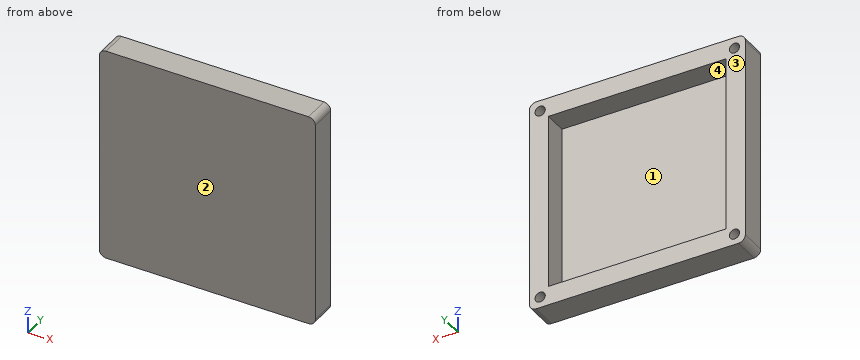
from build123d import *

# Parameters (mm, degrees)
SKETCH1_W           = 63.5
SKETCH1_H           = 63.5
BOSS_EXTRUDE1_DEPTH = 7.8
SKETCH2_W           = 52.2
SKETCH2_H           = 52.2
CUT_EXTRUDE1_DEPTH  = 6.8
SKETCH3_R           = 1.5
CUT_EXTRUDE2_DEPTH  = 7.5
FILLET1_R           = 2


with BuildPart() as part:
    # Sketch1 → Boss-Extrude1 (new body)
    with BuildSketch(Plane(origin=(0, 0, 0), x_dir=(1, 0, 0), z_dir=(0, 1, 0))):
        with Locations((31.75, 31.75)):
            Rectangle(SKETCH1_W, SKETCH1_H)
    extrude(amount=BOSS_EXTRUDE1_DEPTH)

    # Sketch2 → Cut-Extrude1 (cut)
    with BuildSketch(Plane(origin=(0, 7.8, 0), x_dir=(1, 0, 0), z_dir=(0, 1, 0))):
        with Locations((31.75, 31.75)):
            Rectangle(SKETCH2_W, SKETCH2_H)
    extrude(amount=-CUT_EXTRUDE1_DEPTH, mode=Mode.SUBTRACT)

    # Sketch3 → Cut-Extrude2 (cut)
    with BuildSketch(Plane(origin=(0, 7.8, 0), x_dir=(1, 0, 0), z_dir=(0, 1, 0))):
        with Locations(Location((3.2, 3.2, 0), (0, 0, 270))):
            Circle(SKETCH3_R)
        with Locations(Location((3.2, 60.3, 0), (0, 0, 270))):
            Circle(SKETCH3_R)
        with Locations(Location((60.3, 60.3, 0), (0, 0, 270))):
            Circle(SKETCH3_R)
        with Locations(Location((60.3, 3.2, 0), (0, 0, 270))):
            Circle(SKETCH3_R)
    extrude(amount=-CUT_EXTRUDE2_DEPTH, mode=Mode.SUBTRACT)

    # Fillet1
    fillet1_edges = [part.edges().sort_by_distance(p)[0] for p in [
        (0, 3.9, -63.5),
        (63.5, 3.9, -63.5),
        (63.5, 3.9, 0),
        (0, 3.9, 0),
    ]]
    fillet(fillet1_edges, radius=FILLET1_R)


solid = part.part
Build history of the part. All positions in model axes, mm. Face numbers are marked on the shaded views. A direction names the side the tool comes from. Coordinates: 2 decimals unless noted, no trailing zeros. Order: outer loops, then holes, each group sorted by start corner. A loop starts at its lowest first (then second) coordinate and runs counter-clockwise, first axis right, second up. Notation, with made-up numbers: (35, -21.75) - (42, -21.75) arc R20 ccw to (42, -2.75) - close; hole circle Ø3 at (45, -13). An arc over 180 degrees is marked (long way). Write item = value, one per line. Start each with the question number.
1) Saw through at A-A on z = -22.5. Write the cut outline in (x, y), then the cut area to 3 significant figures.
2) Flat gauge pins, fed straight in: pin 1 Ø2.5 at (x, z) = (60.5, -3) entering from +Y; pin 2 Ø0.9 at (x, z) = (2.5, -3.5) entering from +Y. Where does each tip first touch, or does it go through?
3) Saw through at B-B on y = 2.75. Write the cut outline in (x, z), then the cut area to 3 significant figures.
4) Wall check: line 1 along X through (y, z) = (5.5, -3.2); line 2 along X through (y, z) = (7.75, -46); line 3 along Z through (x, y) = (33.5, 5). Give the ranges that are in metal, low to high. Write a range as from..to.
5) Two-plate mould, pull along X, no slides. Class the marked faces 3 and 4: pulls with the +X half, pulls with the -X half, needs draft (parallel to the pull), parting line crosses it, or undercut.
6) Saw through at C-C on x = 7. Write the cut outline in (y, z), then the cut area to 3 significant figures.
7) Saw through at D-D on x = 60.3. Write the cut outline in (y, z), then the cut area to 3 significant figures.
8) 3-axis set-ups, long thin cutter, end or side, ignore diameter. For the marked faces 1 and 2: which of +Z, -Z, +X, -X, +Y, -Y reach the whole face in a straight line?
From the geometry:
q1.outline = (0, 0) - (63.5, 0) - (63.5, 7.8) - (57.85, 7.8) - (57.85, 1) - (5.65, 1) - (5.65, 7.8) - (0, 7.8) - close
q1.area = 140 mm^2
q2.pin_1 = 7.8
q2.pin_2 = 0.3
q3.outline = (0, -61.5) arc R2 ccw to (2, -63.5) - (61.5, -63.5) arc R2 ccw to (63.5, -61.5) - (63.5, -2) arc R2 ccw to (61.5, 0) - (2, 0) arc R2 ccw to (0, -2) - close; hole circle Ø3 at (3.2, -60.3); hole circle Ø3 at (3.2, -3.2); hole (5.65, -57.85) - (57.85, -57.85) - (57.85, -5.65) - (5.65, -5.65) - close; hole circle Ø3 at (60.3, -60.3); hole circle Ø3 at (60.3, -3.2)
q3.area = 1,280 mm^2
q4.line_1 = 0..1.7, 4.7..58.8, 61.8..63.5
q4.line_2 = 0..5.65, 57.85..63.5
q4.line_3 = -63.5..-57.85, -5.65..0
q5.face_3 = needs draft
q5.face_4 = undercut
q6.outline = (0, -63.5) - (7.8, -63.5) - (7.8, -57.85) - (1, -57.85) - (1, -5.65) - (7.8, -5.65) - (7.8, 0) - (0, 0) - close
q6.area = 140 mm^2
q7.outline = (0, -63.5) - (7.8, -63.5) - (7.8, -61.8) - (0.3, -61.8) - (0.3, -58.8) - (7.8, -58.8) - (7.8, -4.7) - (0.3, -4.7) - (0.3, -1.7) - (7.8, -1.7) - (7.8, 0) - (0, 0) - close
q7.area = 450 mm^2
q8.face_1 = +Y
q8.face_2 = +Z, -Z, +X, -X, -Y
